from build123d import *
from OCP.BRepFilletAPI import BRepFilletAPI_MakeChamfer

# Parameters (mm, degrees)
ESBO_O1_W                = 0.64
ESBO_O1_H                = 5.6
RESSALTO_EXTRUS_O1_DEPTH = 0.32
ESBO_O2_W                = 2.54
ESBO_O2_H                = 2.54
RESSALTO_EXTRUS_O2_DEPTH = 1.27
RESSALTO_EXTRUS_O3_DEPTH = 0.32
FILETE1_R                = 0.2
FILETE2_R                = 0.6
CHANFRO1_SIZE            = 0.15
CHANFRO1_SIZE2           = 0.26
CHANFRO2_SIZE            = 0.26
CHANFRO2_SIZE2           = 0.15
CHANFRO3_SIZE            = 0.25


with BuildPart() as part:
    # Esboço1 → Ressalto-extrusão1 (new, symmetric)
    with BuildSketch(Plane.XY):
        with Locations((0, 3)):
            Rectangle(ESBO_O1_W, ESBO_O1_H)
    extrude(amount=RESSALTO_EXTRUS_O1_DEPTH, both=True)

    # Esboço2 → Ressalto-extrusão2 (add, symmetric)
    with BuildSketch(Plane.XY):
        with Locations((0, 1.47)):
            Rectangle(ESBO_O2_W, ESBO_O2_H)
    extrude(amount=RESSALTO_EXTRUS_O2_DEPTH, both=True)

    # Esboço3 → Ressalto-extrusão3 (add, symmetric)
    with BuildSketch(Plane.XY):
        Polygon((0.32, 0.2), (-0.32, 0.2), (-0.32, -1.62), (6.7, -1.62), (6.7, -0.98), (0.32, -0.98), align=None)
    extrude(amount=RESSALTO_EXTRUS_O3_DEPTH, both=True)

    # Filete1
    filete1_edges = [part.edges().sort_by_distance(p)[0] for p in [
        (0.32, -0.98, 0),
    ]]
    fillet(filete1_edges, radius=FILETE1_R)

    # Filete2
    filete2_edges = [part.edges().sort_by_distance(p)[0] for p in [
        (-0.32, -1.62, 0),
    ]]
    fillet(filete2_edges, radius=FILETE2_R)

    # Chanfro1
    chanfro1_edges = [part.edges().sort_by_distance(p)[0] for p in [
        (0, 5.8, 0.32),
        (0, 5.8, -0.32),
        (-0.32, 5.8, 0),
        (0.32, 5.8, 0),
    ]]
    chanfro1_side = [part.faces().sort_by_distance(p)[0] for p in [
        (0, 5.8, 0),
    ]]
    chamfer(chanfro1_edges, length=CHANFRO1_SIZE, length2=CHANFRO1_SIZE2, reference=chanfro1_side[0])

    # Chanfro2: one chamfer whose edges measure the first distance from different faces: ONE call of the kernel's chamfer builder (chamfer() names one face for all edges)
    chanfro2_edges_1 = [part.edges().sort_by_distance(p)[0] for p in [
        (6.7, -1.3, 0.32),
    ]]
    chanfro2_side_1 = [part.faces().sort_by_distance(p)[0] for p in [
        (2.770539373, -1.16393397, 0.32),
    ]]
    chanfro2_edges_2 = [part.edges().sort_by_distance(p)[0] for p in [
        (6.7, -1.62, 0),
    ]]
    chanfro2_side_2 = [part.faces().sort_by_distance(p)[0] for p in [
        (3.49, -1.62, 0),
    ]]
    chanfro2_edges_3 = [part.edges().sort_by_distance(p)[0] for p in [
        (6.7, -0.98, 0),
    ]]
    chanfro2_side_3 = [part.faces().sort_by_distance(p)[0] for p in [
        (3.61, -0.98, 0),
    ]]
    chanfro2_edges_4 = [part.edges().sort_by_distance(p)[0] for p in [
        (6.7, -1.3, -0.32),
    ]]
    chanfro2_side_4 = [part.faces().sort_by_distance(p)[0] for p in [
        (2.770539373, -1.16393397, -0.32),
    ]]
    chanfro2 = BRepFilletAPI_MakeChamfer(part.part.solid().wrapped)
    for e in chanfro2_edges_1:
        chanfro2.Add(CHANFRO2_SIZE, CHANFRO2_SIZE2, e.wrapped, chanfro2_side_1[0].wrapped)  # the first distance lies on this face
    for e in chanfro2_edges_2:
        chanfro2.Add(CHANFRO2_SIZE, CHANFRO2_SIZE2, e.wrapped, chanfro2_side_2[0].wrapped)  # the first distance lies on this face
    for e in chanfro2_edges_3:
        chanfro2.Add(CHANFRO2_SIZE, CHANFRO2_SIZE2, e.wrapped, chanfro2_side_3[0].wrapped)  # the first distance lies on this face
    for e in chanfro2_edges_4:
        chanfro2.Add(CHANFRO2_SIZE, CHANFRO2_SIZE2, e.wrapped, chanfro2_side_4[0].wrapped)  # the first distance lies on this face
    add(Compound.cast(chanfro2.Shape()), mode=Mode.REPLACE)

    # Chanfro3
    chanfro3_edges = [part.edges().sort_by_distance(p)[0] for p in [
        (0, 0.2, -1.27),
        (-1.27, 0.2, 0),
        (0, 2.74, -1.27),
        (1.27, 2.74, 0),
        (-1.27, 1.47, -1.27),
        (-1.27, 2.74, 0),
        (1.27, 1.47, -1.27),
        (1.27, 0.2, 0),
        (-1.27, 1.47, 1.27),
        (0, 0.2, 1.27),
        (1.27, 1.47, 1.27),
        (0, 2.74, 1.27),
    ]]
    chamfer(chanfro3_edges, length=CHANFRO3_SIZE)


solid = part.part
Design review of the part built by this model. Coordinates are the model's own, in mm. A direction names the side the tool comes from. Round coordinates to 2 decimals unless told otherwise and drop trailing zeros. Order: outer loops, then holes, each group sorted by start corner. A loop starts at its lowest first (then second) coordinate and runs counter-clockwise, first axis right, second up. Notation, with made-up numbers: M 14.5,-32.5 L 53.5,-32.5 A15 ccw 53.5,-10.5 Z; hole C 25,-29.75 d8. An arc over 180 degrees is marked long. Answer as CSV lines item,"result". Start each with the question number.
1) The part is to be moulded in two halves that separate along Y. For faces 1 (the face through (0, 2.74, 0.5)), 2 (the face through (-1.27, 1, 0)), 3 (the face through (0, 0.2, 0.5)), say which applies: +Y half, -Y half, draft (parallel to the pull), parting line (faces both ways), or undercut.
2) Add section A-A (y = 2). Give the boundary of the cut face in (x, z).
3) Add section D-D (y = 3.25). Give the boundary of the cut face in (x, z), then the cut area to 3 significant figures.
4) Tool access review of faces 4 (the face through (2.3, -1.3, -0.32)), 5 (the face through (2.3, -1.3, 0.32)), 6 (the face through (1.27, 1, 0)): name each direction out of +Z, -Z, +X, -X, +Y, -Y from which nothing blocks a thin tool from reaching the whole face with its end or side.
5) For pin 1 Ø0.5 at (x, y) = (0, 4) entering from -Z; pin 2 Ø0.7 at (x, y) = (0, 4) entering from +Z; pin 3 Ø1 at (x, z) = (0.5, 0.5) entering from +Y; pin 4 Ø0.5 at (y, z) = (3.5, 0) entering from +X, all flat-tipped, find the tip position at first contact; note any pin that passes through.
6) Wall thickness on line 1 along Y through (x, z) = (0.5, -0.9); line 2 along X through (y, z) = (0.75, 0.75); line 3 along X through (y, z) = (3.5, 0.25): over which ranges is each line inside the solid? List them lowest first. Write a range as [from, to].
7) Add section B-B (z = -0.55). Give the boundary of the cut face in (x, y).
8) Add section C-C (x = 5.5). Give the boundary of the cut face in (y, z).
Resolved:
1,face 1,"+Y half"
1,face 2,"draft"
1,face 3,"undercut"
2,outline,"M -1.27,-1.02 L -1.02,-1.27 L 1.02,-1.27 L 1.27,-1.02 L 1.27,1.02 L 1.02,1.27 L -1.02,1.27 L -1.27,1.02 Z"
3,outline,"M -0.32,-0.32 L 0.32,-0.32 L 0.32,0.32 L -0.32,0.32 Z"
3,area,"0.410 mm^2"
4,face 4,"-Z, +X, -X, -Y"
4,face 5,"+Z, +X, -X, -Y"
4,face 6,"+Z, -Z, +X, +Y"
5,pin 1,"z = -0.32"
5,pin 2,"z = 0.32"
5,pin 3,"y = 5.8"
5,pin 4,"x = 0.32"
6,line 1,"[0.2, 2.74]"
6,line 2,"[-1.27, 1.27]"
6,line 3,"[-0.32, 0.32]"
7,outline,"M -1.27,0.45 L -1.02,0.2 L 1.02,0.2 L 1.27,0.45 L 1.27,2.49 L 1.02,2.74 L -1.02,2.74 L -1.27,2.49 Z"
8,outline,"M -1.62,-0.32 L -0.98,-0.32 L -0.98,0.32 L -1.62,0.32 Z"
